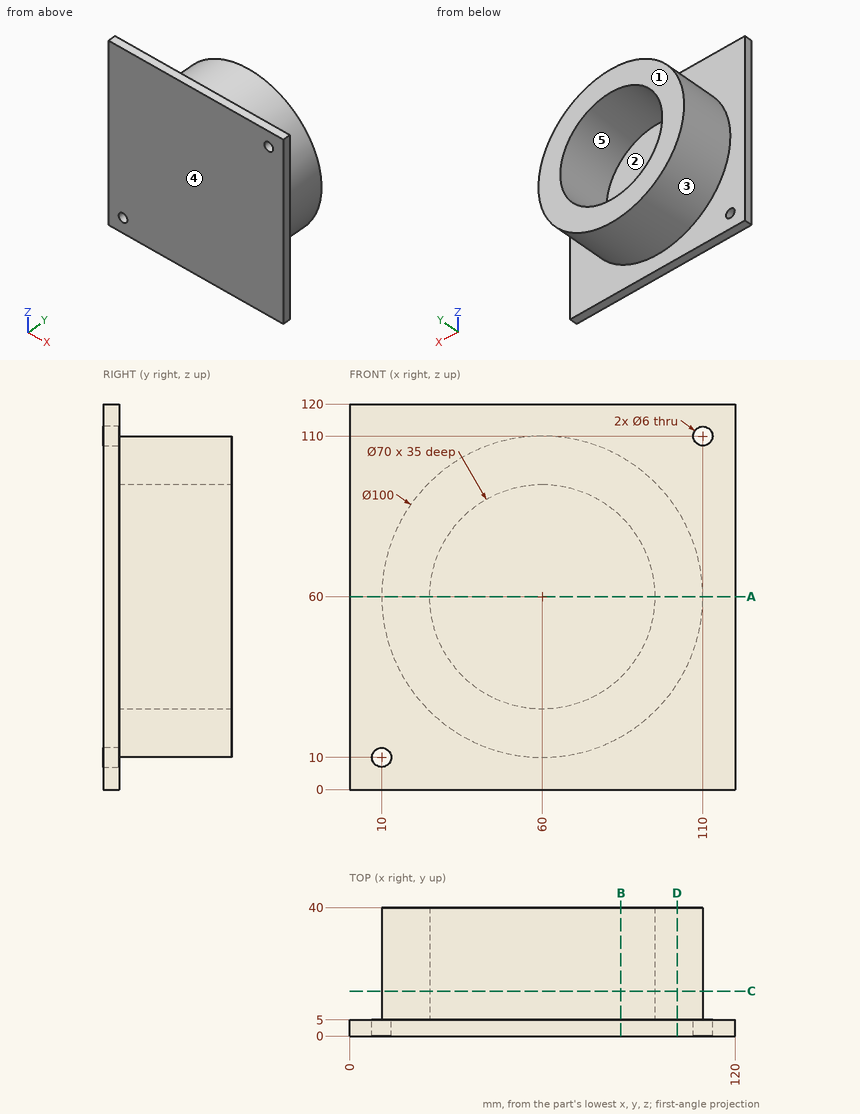
Input: dimensioned drawing with shaded views. Units: mm. Origin: part minimum x, y, z. A direction names the side the tool comes from. Round coordinates to 2 decimals unless told otherwise and drop trailing zeros. Loops run counter-clockwise (first coordinate to the right, second up) from the corner with the lowest first, then second, coordinate; pieces in that order, holes last. Notation, with made-up numbers: (-23, 66) -> (-13, 66) arc R17 cw to (-13, 83) -> close; hole circle Ø10 at (72, 30). An arc over 180 degrees is marked (long way). Answer as a JSON object with one key per item and string values. Group by question number.
1) Pin query (flat end, axial travel): pin 1 (1 mm diameter, centred on y = 11, z = 43.5, fed in from +X); pin 2 (1.5 mm diameter, centred on x = 51, z = 44, fed in from +Y); pin 3 (2 mm diameter, centred on x = 16.5, y = 17.5, fed in from +Z). Return the tip coordinate at first contact, or that it passes through.
2) Section query B-B on x = 84.5. Output: boundary loops of the cut face in (y, z) (3 decimals), plus the area to 3 significant figures.
3) Section query A-A on z = 60. Output: boundary loops of the cut face in (x, y).
4) Section query D-D on x = 102. Output: boundary loops of the cut face in (y, z), plus the area to 3 significant figures.
5) Section query C-C on y = 14. Output: boundary loops of the cut face in (x, z), plus the area to 3 significant figures.
6) Ray query, L1, parallel to X at y = 2, z = 10; L2, parallel to X at y = 3.65, z = 110; L3, parallel to Y at x = 113, z = 104. Return the intervals inside material, ascending.
7) Reachability of the marked faces 4 and 5 from +Z, -Z, +X, -X, +Y, -Y: full face, straight path, thin tool, end or side. Return the list, or none.
8) Draft query along X for the marked faces 1, 2 and 3. Return one class per face: +X half, -X half, draft (parallel to the pull), parting line (faces both ways), or undercut.
Reply:
{
 "1": {"pin 1": "stops at x = 107.37", "pin 2": "stops at y = 5", "pin 3": "stops at z = 86.34"},
 "2": {"outline": "(0, 0) -> (5, 0) -> (5, 16.414) -> (40, 16.414) -> (40, 35.005) -> (5, 35.005) -> (5, 84.995) -> (40, 84.995) -> (40, 103.586) -> (5, 103.586) -> (5, 120) -> (0, 120) -> close", "area": "1,900 mm2"},
 "3": {"outline": "(0, 0) -> (120, 0) -> (120, 5) -> (110, 5) -> (110, 40) -> (95, 40) -> (95, 5) -> (25, 5) -> (25, 40) -> (10, 40) -> (10, 5) -> (0, 5) -> close"},
 "4": {"outline": "(0, 0) -> (5, 0) -> (5, 32.87) -> (40, 32.87) -> (40, 87.13) -> (5, 87.13) -> (5, 120) -> (0, 120) -> close", "area": "2,500 mm2"},
 "5": {"outline": "circle Ø100 at (60, 60); hole circle Ø70 at (60, 60)", "area": "4,010 mm2"},
 "6": {"L1": "x = 0 to 7, 13 to 120", "L2": "x = 0 to 107, 113 to 120", "L3": "y = 0 to 5"},
 "7": {"face 4": "+Z, -Z, +X, -X, -Y", "face 5": "+Y"},
 "8": {"face 1": "draft", "face 2": "undercut", "face 3": "parting line"}
}
